For this review, take the finished solid that the model builds, in its own axes (mm). Coordinates: 2 decimals unless noted, no trailing zeros. Write each loop counter-clockwise with the first axis right and the second up, starting at its lowest first coordinate (ties: lowest second). Pieces come first, ordered by that corner, then holes. Notation, with made-up numbers: (69.25, 35.5) - (84.25, 35.5) arc R32 ccw to (84.25, 62.5) - close; hole circle Ø9 at (-24.75, 48.5). An arc over 180 degrees is marked (long way). Use one line per item in the form item = value. Start each with the question number.
1) We need section A-A (x = 7). Give the boundary of the cut face in (y, z).
2) For L1, parallel to Y at x = 11, z = 1.4; L2, parallel to X at y = 38, z = 2.95, list the stretches that pass through material, from the lowest coordinate up. Write a range as from..to.
3) We need section B-B (y = 41). Give the boundary of the cut face in (x, z), plus the area to 3 significant figures.
4) We need section C-C (z = 4.8). Give the boundary of the cut face in (x, y), plus the area to 3 significant figures.
5) Insertion check: P1, Ø3, axis at y = 18.5, z = 3.5, coming from the +X side; P2, Ø3, axis at y = 38.5, z = 2.5, coming from the -X side. Each pin has a flat end and moves straight along its axis. Give the tip position at first contact, or say it passes through.
```python
from build123d import *

# Parameters (mm, degrees)
BOX002_W     = 25
BOX002_H     = 50
BOX002_DEPTH = 10
BOX003_W     = 25
BOX003_H     = 50
BOX003_DEPTH = 10
BOX001_W     = 14
BOX001_H     = 50
BOX001_DEPTH = 10
BOX_W        = 70
BOX_H        = 60
BOX_DEPTH    = 6


with BuildPart() as cube002:
    # Box002 → Box002 (new body)
    with BuildSketch(Plane(origin=(-2, 5, -1), x_dir=(1, 0, 0), z_dir=(0, 0, 1))):
        with Locations((12.5, 25)):
            Rectangle(BOX002_W, BOX002_H)
    extrude(amount=BOX002_DEPTH)


with BuildPart() as cube003:
    # Box003 → Box003 (new body)
    with BuildSketch(Plane(origin=(47, 5, -1), x_dir=(1, 0, 0), z_dir=(0, 0, 1))):
        with Locations((12.5, 25)):
            Rectangle(BOX003_W, BOX003_H)
    extrude(amount=BOX003_DEPTH)


with BuildPart() as cube001:
    # Box001 → Box001 (new body)
    with BuildSketch(Plane(origin=(28, 5, -1), x_dir=(1, 0, 0), z_dir=(0, 0, 1))):
        with Locations((7, 25)):
            Rectangle(BOX001_W, BOX001_H)
    extrude(amount=BOX001_DEPTH)


with BuildPart() as cut002:
    # Box → Box (new body)
    with BuildSketch(Plane.XY):
        with Locations((35, 30)):
            Rectangle(BOX_W, BOX_H)
    extrude(amount=BOX_DEPTH)

    # Cut: cut Cube001
    add(cube001.part, mode=Mode.SUBTRACT)

    # Cut001: cut Cube003
    add(cube003.part, mode=Mode.SUBTRACT)

    # Cut002: cut Cube002
    add(cube002.part, mode=Mode.SUBTRACT)


solid = cut002.part
```
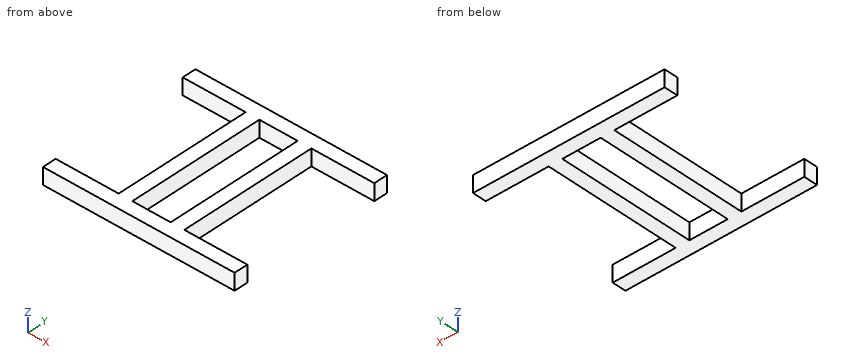
Determined:
q1.outline = (0, 0) - (5, 0) - (5, 6) - (0, 6) - close; (55, 0) - (60, 0) - (60, 6) - (55, 6) - close
q2.L1 = 0..5, 55..60
q2.L2 = 23..28, 42..47
q3.outline = (23, 0) - (28, 0) - (28, 6) - (23, 6) - close; (42, 0) - (47, 0) - (47, 6) - (42, 6) - close
q3.area = 60.0 mm²
q4.outline = (0, 0) - (70, 0) - (70, 5) - (47, 5) - (47, 55) - (70, 55) - (70, 60) - (0, 60) - (0, 55) - (23, 55) - (23, 5) - (0, 5) - close; hole (28, 5) - (42, 5) - (42, 55) - (28, 55) - close
q4.area = 1,200 mm²
q5.P1 = 47
q5.P2 = 23
